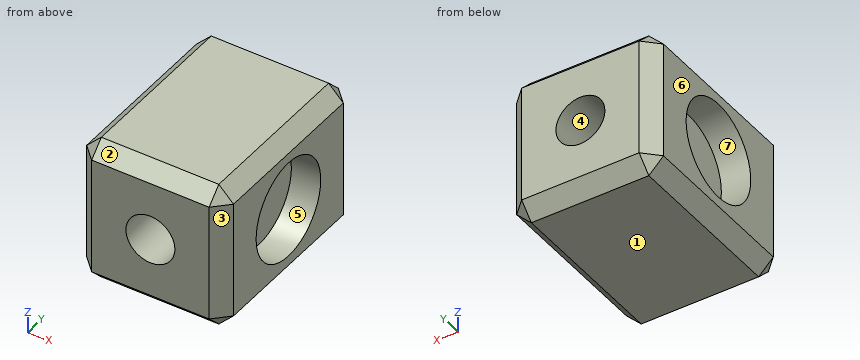
from build123d import *

# Parameters (mm, degrees)
SKETCH1_W           = 38.1
SKETCH1_H           = 38.1
SKETCH1_R           = 6.35
BOSS_EXTRUDE1_DEPTH = 50.8
CUT_EXTRUDE1_START  = 19.05
SKETCH2_R           = 12.7
CUT_EXTRUDE1_DEPTH  = 7.62
CUT_EXTRUDE2_START  = -11.43
SKETCH2_2_R         = 12.7
CUT_EXTRUDE2_DEPTH  = 7.62
CHAMFER1_SIZE       = 3.81


with BuildPart() as part:
    # Sketch1 → Boss-Extrude1 (new body)
    with BuildSketch(Plane(origin=(0, 0, 0), x_dir=(1, 0, 0), z_dir=(0, 1, 0))):
        Rectangle(SKETCH1_W, SKETCH1_H)
        with Locations(Location((0, 0, 0), (0, 0, 270))):
            Circle(SKETCH1_R, mode=Mode.SUBTRACT)
    extrude(amount=BOSS_EXTRUDE1_DEPTH)

    # Sketch2 → Cut-Extrude1 (cut)
    with BuildSketch(Plane(origin=(0, 0, 0), x_dir=(0, 0, -1), z_dir=(1, 0, 0)).offset(CUT_EXTRUDE1_START)):
        with Locations((0, 25.4)):
            Circle(SKETCH2_R)
    extrude(amount=-CUT_EXTRUDE1_DEPTH, mode=Mode.SUBTRACT)

    # Sketch2<2> → Cut-Extrude2 (cut)
    with BuildSketch(Plane(origin=(0, 0, 0), x_dir=(0, 0, -1), z_dir=(1, 0, 0)).offset(CUT_EXTRUDE2_START)):
        with Locations((0, 25.4)):
            Circle(SKETCH2_2_R)
    extrude(amount=-CUT_EXTRUDE2_DEPTH, mode=Mode.SUBTRACT)

    # Chamfer1
    chamfer1_edges = [part.edges().sort_by_distance(p)[0] for p in [
        (-19.05, 50.8, 0),
        (0, 50.8, 19.05),
        (19.05, 50.8, 0),
        (0, 0, 19.05),
        (-19.05, 0, 0),
        (0, 0, -19.05),
        (19.05, 0, 0),
        (19.05, 25.4, 19.05),
        (-19.05, 25.4, 19.05),
        (-19.05, 25.4, -19.05),
        (19.05, 25.4, -19.05),
        (0, 50.8, -19.05),
    ]]
    chamfer(chamfer1_edges, length=CHAMFER1_SIZE)


solid = part.part
Here's how the part is built. I have some questions about the finished solid (model axes, mm). Face numbers are marked on the shaded views. A direction names the side the tool comes from. Round coordinates to 2 decimals unless told otherwise and drop trailing zeros. Order: outer loops, then holes, each group sorted by start corner. A loop starts at its lowest first (then second) coordinate and runs counter-clockwise, first axis right, second up. Notation, with made-up numbers: (-32.5, -11) -> (6.5, -11) arc R6 ccw to (6.5, -5) -> close; hole circle Ø6 at (-40, 57.5). An arc over 180 degrees is marked (long way). Return JSON: item names as keys, results as strings.
Q1. Which directions (+Z, -Z, +X, -X, +Y, -Y) give clear straight access to the entire face, cutting with the end or side of a thin tool? Please do the marked faces 5, 6 and 7.
Filled sheet:
{"face 5": "+X", "face 6": "+Z, -Z, -X, +Y, -Y", "face 7": "-X"}
Q2. If we section it at A-A on x = 16.5: List the corners of the cut face in (y, z) for me.
Filled sheet:
{"outline": "(1.26, -15.24) -> (3.81, -17.79) -> (46.99, -17.79) -> (49.54, -15.24) -> (49.54, 15.24) -> (46.99, 17.79) -> (3.81, 17.79) -> (1.26, 15.24) -> close; hole circle Ø25.4 at (25.4, 0)"}
Q3. If we section it at C-C on y = 25.4: List the corners of the cut face in (x, z) for me, plus the area to 3 significant figures.
Filled sheet:
{"outline": "(-19.05, -15.24) -> (-15.24, -19.05) -> (15.24, -19.05) -> (19.05, -15.24) -> (19.05, -12.7) -> (11.43, -12.7) -> (11.43, 12.7) -> (19.05, 12.7) -> (19.05, 15.24) -> (15.24, 19.05) -> (-15.24, 19.05) -> (-19.05, 15.24) -> (-19.05, 12.7) -> (-11.43, 12.7) -> (-11.43, -12.7) -> (-19.05, -12.7) -> close; hole circle Ø12.7 at (0, 0)", "area": "909 mm^2"}
Q4. If we mould it in two halves opening along Z, with no side actions, what happens to the marked faces 1, 2, 3 and 4? For each: released by +Z, released by -Z, zero draft, split by the parting line, or undercut.
Filled sheet:
{"face 1": "released by -Z", "face 2": "released by +Z", "face 3": "zero draft", "face 4": "undercut"}
Q5. If we section it at B-B on z = 0: List the corners of the cut face in (x, y) for me.
Filled sheet:
{"outline": "(-19.05, 3.81) -> (-15.24, 0) -> (-6.35, 0) -> (-6.35, 50.8) -> (-15.24, 50.8) -> (-19.05, 46.99) -> (-19.05, 38.1) -> (-11.43, 38.1) -> (-11.43, 12.7) -> (-19.05, 12.7) -> close; (6.35, 0) -> (15.24, 0) -> (19.05, 3.81) -> (19.05, 12.7) -> (11.43, 12.7) -> (11.43, 38.1) -> (19.05, 38.1) -> (19.05, 46.99) -> (15.24, 50.8) -> (6.35, 50.8) -> close"}
Q6. For pin 1 Ø8 at (y, z) = (23, -10) entering from +X; pin 2 Ø12.5 at (y, z) = (27, 2) entering from -X; pin 3 Ø10 at (x, z) = (0, 0) entering from +Y; pin 4 Ø20.5 at (y, z) = (25.4, 0) entering from +X, each with a flat end and sliding along its axis, tell me the tip position at first contact or that it passes through.
Filled sheet:
{"pin 1": "stops at x = 19.05", "pin 2": "stops at x = -11.43", "pin 3": "passes through", "pin 4": "stops at x = 11.43"}
Q7. If we section it at D-D on x = 0: List the corners of the cut face in (y, z) for me.
Filled sheet:
{"outline": "(0, -15.24) -> (3.81, -19.05) -> (46.99, -19.05) -> (50.8, -15.24) -> (50.8, -6.35) -> (0, -6.35) -> close; (0, 6.35) -> (50.8, 6.35) -> (50.8, 15.24) -> (46.99, 19.05) -> (3.81, 19.05) -> (0, 15.24) -> close"}
Q8. I need wall thicknesses on line 1 along Y through (x, z) = (-13, 0); line 2 along Z through (x, y) = (-14, 25); line 3 along X through (y, z) = (40, 0). Which ranges of each line are inside material? Lowest first, please. Write a range as from..to.
Filled sheet:
{"line 1": "y = 0..12.7, 38.1..50.8", "line 2": "z = -19.05..-12.69, 12.69..19.05", "line 3": "x = -19.05..-6.35, 6.35..19.05"}
